```python
from build123d import *

# Parameters (mm, degrees)
SKETCH2_W               = 45
SKETCH2_H               = 70
SKETCH2_W_2             = 25
SKETCH2_H_2             = 50
BOSS_EXTRUDE2_DEPTH     = 10
CUT_EXTRUDE1_REACH      = 72
BOSS_EXTRUDE3_DEPTH     = 10
SKETCH6_R               = 3.65
BOSS_EXTRUDE4_DEPTH     = 16
BOSS_EXTRUDE5_DEPTH     = 10
BOSS_EXTRUDE8_DEPTH     = 8
SKETCH9_W               = 6
SKETCH9_H               = 16.4
CUT_EXTRUDE2_DEPTH      = 6
CUT_EXTRUDE3_DEPTH      = 15.5
CUT_EXTRUDE3_DEPTH_BACK = 31.5
SKETCH11_W              = 63.799799384
SKETCH11_H              = 31.786722146
CUT_EXTRUDE4_DEPTH      = 77
SKETCH12_R              = 3.65
BOSS_EXTRUDE9_DEPTH     = 21
SKETCH13_R              = 4.85
SKETCH13_R_2            = 3.65
BOSS_EXTRUDE10_DEPTH    = 2
SKETCH14_R              = 4.85
CUT_EXTRUDE6_DEPTH      = 4
CUT_EXTRUDE7_DEPTH      = 7
FILLET1_R               = 1
SKETCH16_R              = 2.575
CUT_EXTRUDE8_DEPTH      = 13.5
CHAMFER1_SIZE           = 0.5
CHAMFER2_SIZE           = 0.2
SKETCH17_R              = 2.4
CUT_EXTRUDE9_DEPTH      = 12
FILLET2_R               = 2


with BuildPart() as part:
    # Sketch2 → Boss-Extrude2 (new body)
    with BuildSketch(Plane.XY):
        with Locations((0, 35)):
            Rectangle(SKETCH2_W, SKETCH2_H)
        with Locations((0, 35)):
            Rectangle(SKETCH2_W_2, SKETCH2_H_2, mode=Mode.SUBTRACT)
    extrude(amount=BOSS_EXTRUDE2_DEPTH)

    # Sketch3 → Cut-Extrude1 (cut, up to next)
    with BuildSketch(Plane(origin=(0, 70, 0), x_dir=(1, 0, 0), z_dir=(0, 1, 0)), mode=Mode.PRIVATE) as cut_extrude1_sk1:
        Polygon((-12, 0), (-12, -4), (-5, -4), (-5, -8), (5, -8), (5, -4), (12, -4), (12, 0), align=None)
    cut_extrude1_tool1 = extrude(cut_extrude1_sk1.sketch, amount=-CUT_EXTRUDE1_REACH, mode=Mode.PRIVATE) & part.part
    add(cut_extrude1_tool1.solids().sort_by_distance((0, 70, 3.176471))[0], mode=Mode.SUBTRACT)

    # Sketch4 → Boss-Extrude3 (add)
    with BuildSketch(Plane(origin=(0, 70, 0), x_dir=(1, 0, 0), z_dir=(0, 1, 0))):
        with BuildLine():
            Line((-12, -10), (12, -10))
            ThreePointArc((12, -10), (7.5, -11.5), (4.8, -15.4))
            ThreePointArc((4.8, -15.4), (0, -19), (-4.8, -15.4))
            ThreePointArc((-4.8, -15.4), (-7.5, -11.5), (-12, -10))
        make_face()
    extrude(amount=-BOSS_EXTRUDE3_DEPTH)

    # Sketch6 → Boss-Extrude4 (add)
    with BuildSketch(Plane(origin=(0, 70, 0), x_dir=(1, 0, 0), z_dir=(0, 1, 0))):
        with Locations((0, -13)):
            Circle(SKETCH6_R)
    extrude(amount=BOSS_EXTRUDE4_DEPTH)

    # Sketch7 → Boss-Extrude5 (add)
    with BuildSketch(Plane.XZ):
        with BuildLine():
            Line((-22.5, 10), (-22.5, 12.456100996))
            Line((-22.5, 12.456100996), (-15.693142744, 14.258664405))
            ThreePointArc((-15.693142744, 14.258664405), (-10.135286431, 15.948047702), (-4.714257706, 18.035206128))
            ThreePointArc((-4.714257706, 18.035206128), (0, 19), (4.714257706, 18.035206128))
            ThreePointArc((4.714257706, 18.035206128), (10.135286431, 15.948047702), (15.693142744, 14.258664405))
            Line((15.693142744, 14.258664405), (22.5, 12.456100996))
            Line((22.5, 12.456100996), (22.5, 10))
            Line((22.5, 10), (-22.5, 10))
        make_face()
    extrude(amount=-BOSS_EXTRUDE5_DEPTH)

    # Sketch8 → Boss-Extrude8 (add, symmetric)
    with BuildSketch(Plane(origin=(0, 0, 0), x_dir=(0, 0, -1), z_dir=(1, 0, 0))):
        Polygon((-19, 66.9), (-23, 66.9), (-23, 50.5), (-19.5, 50.5), (-10, 60), (-10, 66.9), align=None)
    extrude(amount=BOSS_EXTRUDE8_DEPTH, both=True)

    # Sketch9 → Cut-Extrude2 (cut)
    with BuildSketch(Plane.XY.offset(23)):
        with Locations((0, 58.7)):
            Rectangle(SKETCH9_W, SKETCH9_H)
    extrude(amount=-CUT_EXTRUDE2_DEPTH, mode=Mode.SUBTRACT)

    # Sketch10 → Cut-Extrude3 (cut, two sides)
    with BuildSketch(Plane.ZY.offset(8)) as cut_extrude3_sk:
        with BuildLine():
            Line((18.35, 64.4), (18.35, 54.4))
            ThreePointArc((18.35, 54.4), (20, 52.75), (21.65, 54.4))
            Line((21.65, 54.4), (21.65, 64.4))
            ThreePointArc((21.65, 64.4), (20, 66.05), (18.35, 64.4))
        make_face()
    extrude(amount=CUT_EXTRUDE3_DEPTH, mode=Mode.SUBTRACT)
    extrude(cut_extrude3_sk.sketch, amount=-CUT_EXTRUDE3_DEPTH_BACK, mode=Mode.SUBTRACT)

    # Sketch11 → Cut-Extrude4 (cut, through all)
    with BuildSketch(Plane(origin=(0, 10, 0), x_dir=(1, 0, 0), z_dir=(0, 1, 0))):
        with Locations((-0.274859754, -9.346463675)):
            Rectangle(SKETCH11_W, SKETCH11_H)
    extrude(amount=CUT_EXTRUDE4_DEPTH, mode=Mode.SUBTRACT)

    # Sketch12 → Boss-Extrude9 (add)
    with BuildSketch(Plane(origin=(0, 10, 0), x_dir=(1, 0, 0), z_dir=(0, 1, 0))):
        with Locations((0, -13)):
            Circle(SKETCH12_R)
    extrude(amount=BOSS_EXTRUDE9_DEPTH)

    # Sketch13 → Boss-Extrude10 (add)
    with BuildSketch(Plane(origin=(0, 10, 0), x_dir=(1, 0, 0), z_dir=(0, 1, 0))):
        with Locations((0, -13)):
            Circle(SKETCH13_R)
        with Locations((0, -13)):
            Circle(SKETCH13_R_2, mode=Mode.SUBTRACT)
    extrude(amount=BOSS_EXTRUDE10_DEPTH)

    # Sketch14 → Cut-Extrude6 (cut)
    with BuildSketch(Plane(origin=(0, 10, 0), x_dir=(1, 0, 0), z_dir=(0, 1, 0))):
        with BuildLine():
            Line((22.5, -12.456100996), (22.5, 0))
            Line((22.5, 0), (-22.5, 0))
            Line((-22.5, 0), (-22.5, -12.456100996))
            Line((-22.5, -12.456100996), (-15.693142744, -14.258664405))
            ThreePointArc((-15.693142744, -14.258664405), (-10.135286431, -15.948047702), (-4.714257706, -18.035206128))
            ThreePointArc((-4.714257706, -18.035206128), (0, -19), (4.714257706, -18.035206128))
            ThreePointArc((4.714257706, -18.035206128), (10.135286431, -15.948047702), (15.693142744, -14.258664405))
            Line((15.693142744, -14.258664405), (22.5, -12.456100996))
        make_face()
        with Locations((0, -13)):
            Circle(SKETCH14_R, mode=Mode.SUBTRACT)
    extrude(amount=-CUT_EXTRUDE6_DEPTH, mode=Mode.SUBTRACT)

    # Sketch15 → Cut-Extrude7 (cut, through all)
    with BuildSketch(Plane(origin=(0, 6, 0), x_dir=(1, 0, 0), z_dir=(0, 1, 0))):
        Polygon((6, -2.5), (20, -2.5), (20, -10.531966446), (6, -14.239387769), align=None)
        Polygon((-6, -14.239387769), (-6, -2.5), (-20, -2.5), (-20, -10.531966446), align=None)
    extrude(amount=-CUT_EXTRUDE7_DEPTH, mode=Mode.SUBTRACT)

    # Fillet1
    fillet1_edges = [part.edges().sort_by_distance(p)[0] for p in [
        (20, 3, 2.5),
        (20, 3, 10.531966446),
        (6, 3, 14.239387769),
        (6, 3, 2.5),
        (-6, 3, 14.239387769),
        (-20, 3, 10.531966446),
        (-20, 3, 2.5),
        (-6, 3, 2.5),
    ]]
    fillet(fillet1_edges, radius=FILLET1_R)

    # Sketch16 → Cut-Extrude8 (cut)
    with BuildSketch(Plane(origin=(0, 31, 0), x_dir=(1, 0, 0), z_dir=(0, 1, 0))):
        with Locations((0, -13)):
            Circle(SKETCH16_R)
    extrude(amount=-CUT_EXTRUDE8_DEPTH, mode=Mode.SUBTRACT)

    # Chamfer1
    chamfer1_edges = [part.edges().sort_by_distance(p)[0] for p in [
        (-3.65, 31, 13),
    ]]
    chamfer(chamfer1_edges, length=CHAMFER1_SIZE)

    # Chamfer2
    chamfer2_edges = [part.edges().sort_by_distance(p)[0] for p in [
        (-2.575, 31, 13),
    ]]
    chamfer(chamfer2_edges, length=CHAMFER2_SIZE)

    # Sketch17 → Cut-Extrude9 (cut)
    with BuildSketch(Plane(origin=(0, 17.5, 0), x_dir=(1, 0, 0), z_dir=(0, 1, 0))):
        with Locations((0, -13)):
            Circle(SKETCH17_R)
    extrude(amount=-CUT_EXTRUDE9_DEPTH, mode=Mode.SUBTRACT)

    # Fillet2
    fillet2_edges = [part.edges().sort_by_distance(p)[0] for p in [
        (-22.5, 3, 12.456100996),
        (22.5, 3, 12.456100996),
        (-22.5, 3, 0),
        (22.5, 3, 0),
    ]]
    fillet(fillet2_edges, radius=FILLET2_R)


solid = part.part
```
Work out the finished part from the listing and answer in its coordinate system (mm). A direction names the side the tool comes from. Coordinates: 2 decimals unless noted, no trailing zeros. Order: outer loops, then holes, each group sorted by start corner. A loop starts at its lowest first (then second) coordinate and runs counter-clockwise, first axis right, second up. Notation, with made-up numbers: M 20.5,-31.75 L 28.5,-31.75 A8 ccw 28.5,-19.75 Z; hole C -16,7 d5. An arc over 180 degrees is marked long. Use CSV: the item, a comma, the result in double quotes.
1) Section A-A on z = 6 is taken. Write down the section's boundary in (x, y).
Worked out:
outline,"M -22.5,0 L -20,0 L -20,6 L -22.5,6 Z; M -6,0 L 6,0 L 6,6 L -6,6 Z; M 20,0 L 22.5,0 L 22.5,6 L 20,6 Z"
2) Flat-ended cylindrical pins translate along their axes: pin 1 Ø5 at (x, y) = (-1.5, 25.5) entering from -Z; pin 2 Ø9.5 at (x, z) = (9.5, 12.5) entering from +Y; pin 3 Ø10 at (y, z) = (12.5, 14) entering from +X; pin 4 Ø5 at (x, z) = (13.5, 6.5) entering from +Y. Find the tip coordinate at first contact, or state that the pin passes through.
Worked out:
pin 1,"stops at z = 9.35"
pin 2,"stops at y = 12"
pin 3,"stops at x = 4.85"
pin 4,"passes through"
3) Section C-C on y = 27 is taken. Write down the section's boundary in (x, z) (3 decimals), plus the area to 3 significant figures.
Worked out:
outline,"C 0,13 d7.3; hole C 0,13 d5.15"
area,"21.0 mm^2"
4) Consider line 1 (Z direction, x = 0, y = 24.25) (3 decimals); line 2 (Z direction, x = 0, y = 9); line 3 (X direction, y = 20, z = 13) (3 decimals). Determine where each line is inside the solid, lowest interval first. Write a range as [from, to].
Worked out:
line 1,"z = [9.35, 10.425], [15.575, 16.65]"
line 2,"z = [8.15, 10.6], [15.4, 17.85]"
line 3,"x = [-3.65, -2.575], [2.575, 3.65]"
5) Section D-D on z = 3 is taken. Write down the section's boundary in (x, y), plus the area to 3 significant figures.
Worked out:
outline,"M -22.5,0 L -19.87,0 L -19.87,6 L -22.5,6 Z; M -6.13,0 L 6.13,0 L 6.13,6 L -6.13,6 Z; M 19.87,0 L 22.5,0 L 22.5,6 L 19.87,6 Z"
area,"105 mm^2"
6) Section B-B on x = 0 is taken. Write down the section's boundary in (y, z) (3 decimals).
Worked out:
outline,"M 0,0 L 6,0 L 6,8.15 L 12,8.15 L 12,9.35 L 30.5,9.35 L 31,9.85 L 31,10.225 L 30.8,10.425 L 17.5,10.425 L 17.5,10.6 L 5.5,10.6 L 5.5,15.4 L 17.5,15.4 L 17.5,15.575 L 30.8,15.575 L 31,15.775 L 31,16.15 L 30.5,16.65 L 12,16.65 L 12,17.85 L 6,17.85 L 6,19 L 0,19 Z"
7) For faces 1 (the face through (0, 3, 19)), 2 (the face through (-6, 3, 8)), 3 (the face through (1, 12, 9)), determine the directions among +Z, -Z, +X, -X, +Y, -Y from which every point of the face is accessible in a straight line to the end or side of a thin tool.
Worked out:
face 1,"+Z, +Y, -Y"
face 2,"+Y, -Y"
face 3,"+Y"
